```python
from build123d import *

# Parameters (mm, degrees)
SKETCH1_W           = 120
SKETCH1_H           = 200
SKETCH1_R           = 1.3
BOSS_EXTRUDE2_DEPTH = 3
SKETCH4_W           = 3
SKETCH4_H           = 20
CUT_EXTRUDE1_DEPTH  = 3
SKETCH5_W           = 3
SKETCH5_H           = 20
CUT_EXTRUDE2_DEPTH  = 3
SKETCH7_W           = 3
SKETCH7_H           = 20
CUT_EXTRUDE3_DEPTH  = 3
SKETCH8_W           = 3
SKETCH8_H           = 20
CUT_EXTRUDE4_DEPTH  = 3
SKETCH9_W           = 3
SKETCH9_H           = 20
CUT_EXTRUDE5_DEPTH  = 3
SKETCH11_W          = 3
SKETCH11_H          = 20
CUT_EXTRUDE7_DEPTH  = 3
SKETCH12_W          = 3
SKETCH12_H          = 20
CUT_EXTRUDE8_DEPTH  = 3
SKETCH13_W          = 3
SKETCH13_H          = 20
CUT_EXTRUDE9_DEPTH  = 3
SKETCH14_W          = 3
SKETCH14_H          = 20
CUT_EXTRUDE10_DEPTH = 3
SKETCH15_W          = 3
SKETCH15_H          = 20
CUT_EXTRUDE11_DEPTH = 3
SKETCH16_W          = 20
SKETCH16_H          = 3
CUT_EXTRUDE12_DEPTH = 3
SKETCH17_W          = 20
SKETCH17_H          = 3
CUT_EXTRUDE13_DEPTH = 3
SKETCH19_W          = 20
SKETCH19_H          = 3
CUT_EXTRUDE14_DEPTH = 3


with BuildPart() as part:
    # Sketch1 → Boss-Extrude2 (new body)
    with BuildSketch(Plane.XY):
        with Locations((-110, 50)):
            Rectangle(SKETCH1_W, SKETCH1_H)
        with Locations((-135, 130)):
            Circle(SKETCH1_R, mode=Mode.SUBTRACT)
        with Locations((-84.2, 114.8)):
            Circle(SKETCH1_R, mode=Mode.SUBTRACT)
        with Locations((-84.2, 86.9)):
            Circle(SKETCH1_R, mode=Mode.SUBTRACT)
        with Locations((-135, 81.7)):
            Circle(SKETCH1_R, mode=Mode.SUBTRACT)
    extrude(amount=BOSS_EXTRUDE2_DEPTH)

    # Sketch4 → Cut-Extrude1 (cut)
    with BuildSketch(Plane(origin=(-50, 0, 0), x_dir=(0, 0, -1), z_dir=(1, 0, 0))):
        with Locations((-1.5, 140)):
            Rectangle(SKETCH4_W, SKETCH4_H)
    extrude(amount=-CUT_EXTRUDE1_DEPTH, mode=Mode.SUBTRACT)

    # Sketch5 → Cut-Extrude2 (cut)
    with BuildSketch(Plane(origin=(-50, 0, 0), x_dir=(0, 0, -1), z_dir=(1, 0, 0))):
        with Locations((-1.5, 100)):
            Rectangle(SKETCH5_W, SKETCH5_H)
    extrude(amount=-CUT_EXTRUDE2_DEPTH, mode=Mode.SUBTRACT)

    # Sketch7 → Cut-Extrude3 (cut)
    with BuildSketch(Plane(origin=(-50, 0, 0), x_dir=(0, 0, -1), z_dir=(1, 0, 0))):
        with Locations((-1.5, 60)):
            Rectangle(SKETCH7_W, SKETCH7_H)
    extrude(amount=-CUT_EXTRUDE3_DEPTH, mode=Mode.SUBTRACT)

    # Sketch8 → Cut-Extrude4 (cut)
    with BuildSketch(Plane(origin=(-50, 0, 0), x_dir=(0, 0, -1), z_dir=(1, 0, 0))):
        with Locations((-1.5, 20)):
            Rectangle(SKETCH8_W, SKETCH8_H)
    extrude(amount=-CUT_EXTRUDE4_DEPTH, mode=Mode.SUBTRACT)

    # Sketch9 → Cut-Extrude5 (cut)
    with BuildSketch(Plane(origin=(-50, 0, 0), x_dir=(0, 0, -1), z_dir=(1, 0, 0))):
        with Locations((-1.5, -20)):
            Rectangle(SKETCH9_W, SKETCH9_H)
    extrude(amount=-CUT_EXTRUDE5_DEPTH, mode=Mode.SUBTRACT)

    # Sketch11 → Cut-Extrude7 (cut)
    with BuildSketch(Plane.ZY.offset(170)):
        with Locations((1.5, 140)):
            Rectangle(SKETCH11_W, SKETCH11_H)
    extrude(amount=-CUT_EXTRUDE7_DEPTH, mode=Mode.SUBTRACT)

    # Sketch12 → Cut-Extrude8 (cut)
    with BuildSketch(Plane.ZY.offset(170)):
        with Locations((1.5, 100)):
            Rectangle(SKETCH12_W, SKETCH12_H)
    extrude(amount=-CUT_EXTRUDE8_DEPTH, mode=Mode.SUBTRACT)

    # Sketch13 → Cut-Extrude9 (cut)
    with BuildSketch(Plane.ZY.offset(170)):
        with Locations((1.5, 60)):
            Rectangle(SKETCH13_W, SKETCH13_H)
    extrude(amount=-CUT_EXTRUDE9_DEPTH, mode=Mode.SUBTRACT)

    # Sketch14 → Cut-Extrude10 (cut)
    with BuildSketch(Plane.ZY.offset(170)):
        with Locations((1.5, 20)):
            Rectangle(SKETCH14_W, SKETCH14_H)
    extrude(amount=-CUT_EXTRUDE10_DEPTH, mode=Mode.SUBTRACT)

    # Sketch15 → Cut-Extrude11 (cut)
    with BuildSketch(Plane.ZY.offset(170)):
        with Locations((1.5, -20)):
            Rectangle(SKETCH15_W, SKETCH15_H)
    extrude(amount=-CUT_EXTRUDE11_DEPTH, mode=Mode.SUBTRACT)

    # Sketch16 → Cut-Extrude12 (cut)
    with BuildSketch(Plane(origin=(0, -50, 0), x_dir=(-1, 0, 0), z_dir=(0, -1, 0))):
        with Locations((60, -1.5)):
            Rectangle(SKETCH16_W, SKETCH16_H)
    extrude(amount=-CUT_EXTRUDE12_DEPTH, mode=Mode.SUBTRACT)

    # Sketch17 → Cut-Extrude13 (cut)
    with BuildSketch(Plane(origin=(0, -50, 0), x_dir=(-1, 0, 0), z_dir=(0, -1, 0))):
        with Locations((100, -1.5)):
            Rectangle(SKETCH17_W, SKETCH17_H)
    extrude(amount=-CUT_EXTRUDE13_DEPTH, mode=Mode.SUBTRACT)

    # Sketch19 → Cut-Extrude14 (cut)
    with BuildSketch(Plane(origin=(0, -50, 0), x_dir=(-1, 0, 0), z_dir=(0, -1, 0))):
        with Locations((140, -1.5)):
            Rectangle(SKETCH19_W, SKETCH19_H)
    extrude(amount=-CUT_EXTRUDE14_DEPTH, mode=Mode.SUBTRACT)


solid = part.part
```
Geometry check sheet. Reference: the model listing, model coordinates, mm. Give positions to 0.01 mm unless a question says otherwise; leave off trailing zeros. Order: outer loops, then holes, each group sorted by start corner. A loop starts at its lowest first (then second) coordinate and runs counter-clockwise, first axis right, second up. Notation, with made-up numbers: (66.5, -33.5) - (114.5, -33.5) arc R14 cw to (114.5, -9.5) - close; hole circle Ø10 at (37, -8). An arc over 180 degrees is marked (long way). Write item = value, one per line. Start each with the question number.
1) Gauge pin test, flat ends, axial feed: pin 1 Ø0.9 at (x, z) = (-52, 2) entering from +Y; pin 2 Ø0.9 at (y, z) = (-22, 2) entering from +X; pin 3 Ø0.9 at (y, z) = (138.5, 2) entering from -X. Record the tip position at first contact, or that the pin passes through.
2) Section check B-B (z = 1.3). Count the separate pieces of the cut face and the enclosed holes in it, then the cut area to 3 significant figures.
3) Section check A-A (y = 136). Enter the section's corners in (x, z).
4) Scan lines: L1, parallel to Y at x = -84.2, z = 1.5; L2, parallel to Y at x = -135, z = 1.35; L3, parallel to X at y = 81.7, z = 1.2. Record each from-to range of solid material in increasing order.
Geometry check:
q1.pin_1 = 130
q1.pin_2 = -53
q1.pin_3 = -167
q2.separate_pieces = 1
q2.enclosed_holes = 4
q2.area = 23,200 mm2
q3.outline = (-167, 0) - (-53, 0) - (-53, 3) - (-167, 3) - close
q4.L1 = -50 to 85.6, 88.2 to 113.5, 116.1 to 150
q4.L2 = -47 to 80.4, 83 to 128.7, 131.3 to 150
q4.L3 = -170 to -136.3, -133.7 to -50
